```python
from build123d import *

# Parameters (mm, degrees)
F0_R      = 53.381002
F1_DEPTH  = 5
F2_R      = 42.843554
F3_DEPTH  = 5
F4_W      = 10.931604
F4_H      = 106.757529
F5_DEPTH  = 25.4
F5_FACE_W = 10.931604
F5_FACE_H = 106.75753
F6_DEPTH  = 25.4


with BuildPart() as f1:
    # F0 (on Top) → F1 (new body)
    with BuildSketch(Plane.XY):
        Circle(F0_R)
    extrude(amount=F1_DEPTH)

    # F2 (on face) → F3 (cut)
    with BuildSketch(Plane.XY.offset(5)):
        Circle(F2_R)
    extrude(amount=-F3_DEPTH, mode=Mode.SUBTRACT)

    # F4 (on Top) → F5 (join)
    with BuildSketch(Plane.XY):
        with Locations((53.262476, 0.232588)):
            Rectangle(F4_W, F4_H)
    extrude(amount=F5_DEPTH)

    # F5_face (on face) → F6 (cut)
    with BuildSketch(Plane(origin=(53.262476, 0.232588, 25.4), x_dir=(1, 0, 0), z_dir=(0, 0, 1))):
        Rectangle(F5_FACE_W, F5_FACE_H)
    extrude(amount=-F6_DEPTH, mode=Mode.SUBTRACT)


solid = f1.part
```
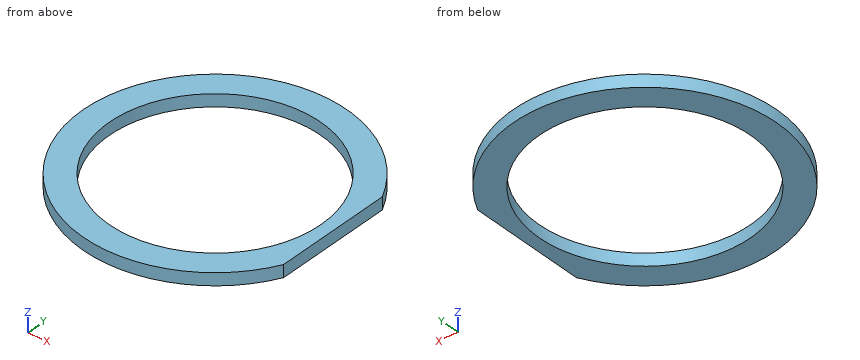
Input: part model. Units: mm. Frame: model coordinates. Round coordinates to 2 decimals unless told otherwise and drop trailing zeros. Order: outer loops, then holes, each group sorted by start corner. A loop starts at its lowest first (then second) coordinate and runs counter-clockwise, first axis right, second up. Notation, with made-up numbers: (-34.75, -22) - (10.25, -22) arc R12 cw to (10.25, -18) - close; hole circle Ø5 at (36.5, 4.25). An arc over 180 degrees is marked (long way). Answer in a Markdown table with one row per item.
Item 1: Line query: line 1 (Y direction, x = 0, z = 4); line 2 (Y direction, x = -14, z = 0.6); line 3 (X direction, y = -36, z = 1.5). Output: solid intervals per line, ascending.
Model answer:
| item | result |
|---|---|
| line 1 | y = -53.38 to -42.84, 42.84 to 53.38 |
| line 2 | y = -51.51 to -40.49, 40.49 to 51.51 |
| line 3 | x = -39.41 to -23.23, 23.23 to 39.41 |
Item 2: Section query A-A (x = 0). Return the cut outline in (y, z), then the cut area to 3 significant figures.
Model answer:
| item | result |
|---|---|
| outline | (-53.38, 0) - (-42.84, 0) - (-42.84, 5) - (-53.38, 5) - close; (42.84, 0) - (53.38, 0) - (53.38, 5) - (42.84, 5) - close |
| area | 105 mm² |
Item 3: Section query B-B (y = 0). Return the cut outline in (x, z).
Model answer:
| item | result |
|---|---|
| outline | (-53.38, 0) - (-42.84, 0) - (-42.84, 5) - (-53.38, 5) - close; (42.84, 0) - (47.8, 0) - (47.8, 5) - (42.84, 5) - close |
Item 4: Pin query (flat end, axial travel): pin 1 (12 mm diameter, centred on x = 30.5, y = 20.5, fed in from -Z); pin 2 (2 mm diameter, centred on x = -23.5, z = 4.5, fed in from +Y); pin 3 (1 mm diameter, centred on x = -4.5, z = 1.5, fed in from -Y); pin 4 (5 mm diameter, centred on x = 21.5, y = -38, fed in from -Z). Return the tip coordinate at first contact, or that it passes through.
Model answer:
| item | result |
|---|---|
| pin 1 | passes through |
| pin 2 | stops at y = 48.41 |
| pin 3 | stops at y = -53.23 |
| pin 4 | stops at z = 0 |
Item 5: Section query C-C (z = 2). Return the cut outline in (x, y).
Model answer:
| item | result |
|---|---|
| outline | (47.8, -23.77) - (47.8, 23.77) arc R53.38 ccw (long way) to start; hole circle Ø85.69 at (0, 0) |
Item 6: Section query D-D (y = 47). Return the cut outline in (x, z), then the cut area to 3 significant figures.
Model answer:
| item | result |
|---|---|
| outline | (-25.31, 0) - (25.31, 0) - (25.31, 5) - (-25.31, 5) - close |
| area | 253 mm² |
